```python
from build123d import *

# Parameters (mm, degrees)
SKETCH1_R           = 3.175
SKETCH1_R_2         = 1.75
SKETCH1_W           = 10
SKETCH1_H           = 5
BOSS_EXTRUDE2_DEPTH = 3.175


with BuildPart() as part:
    # Sketch1 → Boss-Extrude2 (new body)
    with BuildSketch(Plane(origin=(0, 0, 0), x_dir=(1, 0, 0), z_dir=(0, 1, 0))):
        Polygon((0, 0), (139.55, 0), (155.5, 0), (155.5, 145), (139.55, 145), (0, 145), (-15.95, 145), (-15.95, 0), align=None)
        with Locations(Location((15, 130, 0), (0, 0, 270))):
            Circle(SKETCH1_R, mode=Mode.SUBTRACT)
        with Locations(Location((124.55, 130, 0), (0, 0, 90))):
            Circle(SKETCH1_R, mode=Mode.SUBTRACT)
        with Locations(Location((15, 15, 0), (0, 0, 90))):
            Circle(SKETCH1_R, mode=Mode.SUBTRACT)
        with Locations(Location((124.55, 15, 0), (0, 0, 270))):
            Circle(SKETCH1_R, mode=Mode.SUBTRACT)
        with Locations(Location((-5.663, 134.0145, 0), (0, 0, 270))):
            Circle(SKETCH1_R_2, mode=Mode.SUBTRACT)
        with Locations(Location((-5.663, 108.6145, 0), (0, 0, 270))):
            Circle(SKETCH1_R_2, mode=Mode.SUBTRACT)
        with Locations(Location((145.213, 134.0145, 0), (0, 0, 90))):
            Circle(SKETCH1_R_2, mode=Mode.SUBTRACT)
        with Locations(Location((145.213, 108.6145, 0), (0, 0, 90))):
            Circle(SKETCH1_R_2, mode=Mode.SUBTRACT)
        with Locations(Location((145.213, 10.9855, 0), (0, 0, 270))):
            Circle(SKETCH1_R_2, mode=Mode.SUBTRACT)
        with Locations(Location((-5.663, 10.9855, 0), (0, 0, 90))):
            Circle(SKETCH1_R_2, mode=Mode.SUBTRACT)
        with Locations(Location((145.213, 36.3855, 0), (0, 0, 270))):
            Circle(SKETCH1_R_2, mode=Mode.SUBTRACT)
        with Locations(Location((-5.663, 36.3855, 0), (0, 0, 90))):
            Circle(SKETCH1_R_2, mode=Mode.SUBTRACT)
        with Locations((69.775, 127.5)):
            Rectangle(SKETCH1_W, SKETCH1_H, mode=Mode.SUBTRACT)
        with Locations((69.775, 17.5)):
            Rectangle(SKETCH1_W, SKETCH1_H, mode=Mode.SUBTRACT)
    extrude(amount=BOSS_EXTRUDE2_DEPTH)


solid = part.part
```
Part model, mm, in its own coordinate system. Coordinates: 2 decimals unless noted, no trailing zeros. Order: outer loops, then holes, each group sorted by start corner. A loop starts at its lowest first (then second) coordinate and runs counter-clockwise, first axis right, second up. Notation, with made-up numbers: (-4.75, -9) -> (9.25, -9) arc R17 ccw to (9.25, -4) -> close; hole circle Ø10 at (80, -28). An arc over 180 degrees is marked (long way). Put each result on its own line as item: value. Start each with the question number.
(1) Probe line 1 along X through (y, z) = (1.3, -19) (3 decimals); line 2 along X through (y, z) = (2.9, -128) (3 decimals). List the from-to ranges inside material, lowest first. Write a range as [from, to].
(2) Band-saw the part on A-A (x = 15). Give the cut face in (y, z) (3 decimals).
(3) Mould opens along X. For faces 1 (the face through (69, 0, -74)), 2 (the face through (14.05, 1.57, -18.03)) say: pulls with the +X half, pulls with the -X half, needs draft (parallel to the pull), parting line crosses it, or undercut.
Determined:
1. line 1: x = [-15.95, 64.775], [74.775, 155.5]
1. line 2: x = [-15.95, 12.534], [17.466, 64.775], [74.775, 122.084], [127.016, 155.5]
2. outline: (0, -145) -> (3.175, -145) -> (3.175, -133.175) -> (0, -133.175) -> close; (0, -126.825) -> (3.175, -126.825) -> (3.175, -18.175) -> (0, -18.175) -> close; (0, -11.825) -> (3.175, -11.825) -> (3.175, 0) -> (0, 0) -> close
3. face 1: needs draft
3. face 2: undercut
